Part model, mm, in its own coordinate system. Give positions to 0.01 mm unless a question says otherwise; leave off trailing zeros. Order: outer loops, then holes, each group sorted by start corner. A loop starts at its lowest first (then second) coordinate and runs counter-clockwise, first axis right, second up. Notation, with made-up numbers: (-2, 7) - (30, 7) arc R33 ccw to (30, 39) - close; hole circle Ø3 at (53, 44). An arc over 180 degrees is marked (long way). Use a Markdown table: item, result. Add a question column.
from build123d import *

# Parameters (mm, degrees)
F0_R     = 6.35
F1_DEPTH = 18.542
F2_W     = 88.9
F2_H     = 18.542
F3_DEPTH = 25.4


with BuildPart() as f1:
    # F0 (on Top) → F1 (new body)
    with BuildSketch(Plane.XY):
        Polygon((341.138078, 177.8), (-954.261922, 177.8), (-954.261922, -139.7), (-598.661922, -139.7), (-598.661922, -215.9), (-954.261922, -215.9), (-954.261922, -533.4), (341.138078, -533.4), (341.138078, -355.6), (976.138078, -355.6), (976.138078, 0), (341.138078, 0), align=None)
        with Locations((823.738078, -177.8)):
            Circle(F0_R, mode=Mode.SUBTRACT)
    extrude(amount=F1_DEPTH)

    # F2 (on face) → F3 (cut)
    with BuildSketch(Plane.XY.offset(18.542)):
        with Locations((-494.261886, -441.071)):
            Rectangle(F2_W, F2_H)
        with Locations((-494.261886, 85.471)):
            Rectangle(F2_W, F2_H)
        with Locations((-316.461886, -441.071)):
            Rectangle(F2_W, F2_H)
        with Locations((-316.461886, 85.471)):
            Rectangle(F2_W, F2_H)
    extrude(amount=-F3_DEPTH, mode=Mode.SUBTRACT)


solid = f1.part
1. Drill centre lines: probe 1 along Y at (x, z) = (-298, 15.5); probe 2 along Y at (x, z) = (796.5, 6.75); probe 3 along X at (y, z) = (-144, 3). Where is each one in solid material? Low to high. Write a range as [from, to].
2. Pin check, flat tips, straight feed: P1, Ø9.5, axis at y = -161.5, z = 6.5, coming from the -X side; P2, Ø9.5, axis at y = 87, z = 12.5, coming from the +X side. Stop position of each tip, or through.
3. Cut at A-A (x = 661). Write the cut outline in (y, z).
Responses:
| question | item | result |
|---|---|---|
| 1 | probe 1 | y = [-533.4, -450.34], [-431.8, 76.2], [94.74, 177.8] |
| 1 | probe 2 | y = [-355.6, 0] |
| 1 | probe 3 | x = [-598.66, 976.14] |
| 2 | P1 | stops at x = -598.66 |
| 2 | P2 | stops at x = 341.14 |
| 3 | outline | (-355.6, 0) - (0, 0) - (0, 18.54) - (-355.6, 18.54) - close |
